```python
from build123d import *

# Parameters (mm, degrees)
SKETCH011_W             = 160
SKETCH011_H             = 50
SKETCH011_R             = 1.2
SKETCH011_W_2           = 27.5
SKETCH011_H_2           = 31.5
PAD004_DEPTH            = 4
SKETCH012_W             = 151.8
SKETCH012_H             = 41.8
SKETCH012_W_2           = 147.8
SKETCH012_H_2           = 37.8
PAD005_DEPTH            = 30
SKETCH013_W             = 160
SKETCH013_H             = 50
SKETCH013_W_2           = 151.8
SKETCH013_H_2           = 41.8
PAD006_DEPTH            = 20
SKETCH014_W             = 20.2
SKETCH014_H             = 5
POCKET004_DEPTH         = 27
SKETCH027_R             = 1.2
POCKET014_DEPTH         = 160.001
POCKET015_DEPTH         = 30.001
LINEARPATTERN007_COUNT  = 5
LINEARPATTERN007_PITCH  = 7.5
BODY002_PLACEMENT_ANGLE = 180


with BuildPart() as part:
    # Sketch011 → Pad004 (new body)
    with BuildSketch(Plane.YZ):
        with Locations((0, 25)):
            Rectangle(SKETCH011_W, SKETCH011_H)
        with Locations((22, 23.75)):
            Circle(SKETCH011_R, mode=Mode.SUBTRACT)
        with Locations((58, 23.75)):
            Circle(SKETCH011_R, mode=Mode.SUBTRACT)
        with Locations((40, 23.75)):
            Rectangle(SKETCH011_W_2, SKETCH011_H_2, mode=Mode.SUBTRACT)
    extrude(amount=PAD004_DEPTH)

    # Sketch012 → Pad005 (join)
    with BuildSketch(Plane.YZ):
        with Locations((0, 25)):
            Rectangle(SKETCH012_W, SKETCH012_H)
        with Locations((0, 25)):
            Rectangle(SKETCH012_W_2, SKETCH012_H_2, mode=Mode.SUBTRACT)
    extrude(amount=PAD005_DEPTH)

    # Sketch013 → Pad006 (join)
    with BuildSketch(Plane.YZ):
        with Locations((0, 25)):
            Rectangle(SKETCH013_W, SKETCH013_H)
        with Locations((0, 25)):
            Rectangle(SKETCH013_W_2, SKETCH013_H_2, mode=Mode.SUBTRACT)
    extrude(amount=PAD006_DEPTH)

    # Sketch014 (on DatumPlane) → Pocket004 (cut)
    with BuildSketch(Plane.XZ.offset(-80)):
        with Locations((14.1, 43.5)):
            Rectangle(SKETCH014_W, SKETCH014_H)
    extrude(amount=POCKET004_DEPTH, mode=Mode.SUBTRACT)

    # Sketch027 (on DatumPlane) → Pocket014 (cut, through all)
    with BuildSketch(Plane.XZ.offset(-80)):
        with Locations((25, 24)):
            Circle(SKETCH027_R)
    extrude(amount=POCKET014_DEPTH, mode=Mode.SUBTRACT)

    # Sketch028 → Pocket015 (cut, through all)
    with BuildSketch(Plane.YZ):
        with BuildLine():
            Line((6, 11.5), (-64, 11.5))
            ThreePointArc((-64, 11.5), (-65.5, 10), (-64, 8.5))
            Line((6, 8.5), (-64, 8.5))
            ThreePointArc((6, 8.5), (7.5, 10), (6, 11.5))
        make_face()
    pocket015 = extrude(amount=POCKET015_DEPTH, mode=Mode.SUBTRACT)

    # LinearPattern007: Pocket015 ×5
    with Locations(*[(0, 0, i * LINEARPATTERN007_PITCH) for i in range(1, LINEARPATTERN007_COUNT)]):
        add(pocket015, mode=Mode.SUBTRACT)


with BuildPart() as part_1:
    # Body002 placement: moved
    add(part.part.moved(Location((200, 0, -4))).rotate(Axis((200, 0, -4), (0, 0, 1)), BODY002_PLACEMENT_ANGLE))


solid = part_1.part
```
Verification items for the finished model (mm, model axes). A direction names the side the tool comes from. Give positions to 0.01 mm unless a question says otherwise; leave off trailing zeros. Loops run counter-clockwise (first coordinate to the right, second up) from the corner with the lowest first, then second, coordinate; pieces in that order, holes last.
1. Section check D-D, the plane y = -16. Enter the section's corners in (x, z).
2. Set-up check for faces 4 (the flat face through (190, -80, 21)), 5 (the cylindrical face through (198, 65.5, 21)): record each of +Z, -Z, +X, -X, +Y, -Y from which the full face is reachable in a straight line by a thin tool's end or side.
3. Go/stop test with flat-tipped pins: pin 1 Ø5 at (x, y) = (177, -16) entering from +Z; pin 2 Ø3 at (y, z) = (-58, 19.75) entering from -X; pin 3 Ø5 at (x, z) = (175, 25) entering from -Y; pin 4 Ø1.9 at (x, z) = (175, 20) entering from +Y. Record where each tip stops, or that it passes through.
4. Section check C-C, the plane x = 193. Enter the section's corners in (y, z), then the cut area to 3 significant figures.
5. Thickness scan on line 1 (Y direction, x = 190.5, z = 5); line 2 (Y direction, x = 174, z = 2.5); line 3 (Z direction, x = 184, y = 69). Record the ranges inside material, lowest first.
6. Section check B-B, the plane z = 25.5. Enter the section's corners in (x, y), then the cut area to 3 significant figures.
7. Mould release check, pull along Z, two halves, no side actions. Record for faces 1 (the flat face through (175, 1, 0.1)), 2 (the cylindrical face through (198, 65.5, 6)), 3 (the flat face through (180, 6, -1)): released by +Z, released by -Z, zero draft, split by the parting line, or undercut.
8. Section check A-A, the plane y = 27.5. Count the separate pieces of the cut face and the enclosed holes in it, then the cut area to 3 significant figures.
Geometry says:
1. outline: (170, 0.1) - (180, 0.1) - (180, -4) - (200, -4) - (200, 46) - (180, 46) - (180, 41.9) - (170, 41.9) - (170, 39.9) - (196, 39.9) - (196, 2.1) - (170, 2.1) - close
2. face 4: +Z, -Z, +X, -X, -Y
2. face 5: +X, -X
3. pin 1: stops at z = 41.9
3. pin 2: stops at x = 196
3. pin 3: stops at y = -75.9
3. pin 4: passes through
4. outline: (-80, -4) - (80, -4) - (80, 46) - (-80, 46) - (-80, 42) - (-53, 42) - (-53, 39.9) - (73.9, 39.9) - (73.9, 2.1) - (-73.9, 2.1) - (-73.9, 37) - (-80, 37) - close
4. area: 2,340 mm2
5. line 1: y = -80 to -73.9, 73.9 to 80
5. line 2: y = -75.9 to -73.9, 73.9 to 75.9
5. line 3: z = -4 to 2.1, 39.9 to 46
6. outline: (170, -75.9) - (180, -75.9) - (180, -80) - (200, -80) - (200, -53.75) - (196, -53.75) - (196, -73.9) - (170, -73.9) - close; (170, 73.9) - (196, 73.9) - (196, -26.25) - (200, -26.25) - (200, 80) - (180, 80) - (180, 75.9) - (170, 75.9) - close
6. area: 765 mm2
7. face 1: released by -Z
7. face 2: undercut
7. face 3: zero draft
8. separate pieces: 6
8. enclosed holes: 0
8. area: 375 mm2
